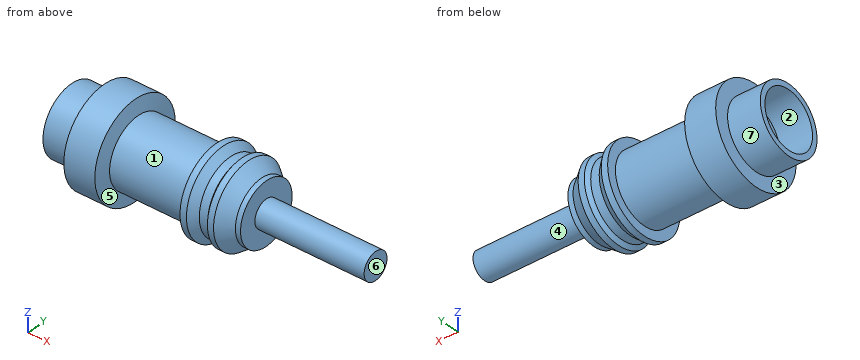
```python
from build123d import *

# Parameters (mm, degrees)
SKETCH_2_R          = 5.2
CUT_EXTRUDE_1_DEPTH = 6
SKETCH_3_R          = 2.5
EXTRUDE_1_DEPTH     = 20


with BuildPart() as part:
    # 草图1 → 旋转1 (revolve)
    with BuildSketch(Plane.XY):
        Polygon((0, 0), (0, 6.2), (6, 6.2), (6, 8.8), (11.676949671, 8.8), (12.2, 6.2), (26.523039375, 6.2), (26.523039375, 7.91006879), (27.695766684, 7.91006879), (29.059190298, 6.725292283), (30.614076117, 6.725292283), (31.1695333, 7.470731504), (32.294644919, 7.470731504), (34.759713658, 5.633908195), (35.7, 5.633908195), (35.7, 0), align=None)
    revolve(axis=Axis((35.7, 0, 0), (-1, 0, 0)))

    # 草图2 → 切除-拉伸1 (cut)
    with BuildSketch(Plane.ZY):
        with Locations(Location((0, 0, 0), (0, 0, 270))):
            Circle(SKETCH_2_R)
    extrude(amount=-CUT_EXTRUDE_1_DEPTH, mode=Mode.SUBTRACT)

    # 草图3 → 凸台-拉伸1 (add)
    with BuildSketch(Plane(origin=(35.7, 0, 0), x_dir=(0, 0, -1), z_dir=(1, 0, 0))):
        with Locations(Location((0, 0, 0), (0, 0, 90))):
            Circle(SKETCH_3_R)
    extrude(amount=EXTRUDE_1_DEPTH)


solid = part.part
```
Verification items for the finished model (mm, model axes). Face numbers are marked on the shaded views. A direction names the side the tool comes from. Give positions to 0.01 mm unless a question says otherwise; leave off trailing zeros. Order: outer loops, then holes, each group sorted by start corner. A loop starts at its lowest first (then second) coordinate and runs counter-clockwise, first axis right, second up. Notation, with made-up numbers: (71, 45) -> (111, 45) arc R16 cw to (111, 67) -> close; hole circle Ø4 at (-20.75, 61). An arc over 180 degrees is marked (long way). Use a Markdown table: item, result.
1) Material ranges on probe 1 along X at (y, z) = (6.75, 2); probe 2 along X at (y, z) = (7.25, -1.25); probe 3 along Z at (x, y) = (2.7, 0), recorded low to high.
Results:
| item | result |
|---|---|
| probe 1 | 6 to 12.03, 26.52 to 28.7, 30.85 to 32.87 |
| probe 2 | 6 to 11.97, 26.52 to 28.33, 31.08 to 32.45 |
| probe 3 | -6.2 to -5.2, 5.2 to 6.2 |
2) Depth check by flat-ended pin: pin 1 Ø4 at (y, z) = (6, 6) entering from -X; pin 2 Ø6 at (x, y) = (24, 2) entering from -Z; pin 3 Ø6 at (y, z) = (-6.5, 5) entering from +X. Enter the tip coordinate at first touch or a pass-through.
Results:
| item | result |
|---|---|
| pin 1 | x = 6 |
| pin 2 | z = -7.9 |
| pin 3 | x = 35.7 |
3) Mould release check, pull along X, two halves, no side actions. Record for the marked faces 1, 2 and 3: pulls with the +X half, pulls with the -X half, needs draft (parallel to the pull), parting line crosses it, or undercut.
Results:
| item | result |
|---|---|
| face 1 | undercut |
| face 2 | needs draft |
| face 3 | pulls with the -X half |
4) Section check B-B, the plane x = 22. Record the boundary of the cut face in (y, z), then the cut area to 3 significant figures.
Results:
| item | result |
|---|---|
| outline | circle Ø12.4 at (0, 0) |
| area | 121 mm² |
5) Tool access check on the marked faces 4, 5, 6 and 7. Record the directions out of +Z, -Z, +X, -X, +Y, -Y that give a thin tool (end or side, any length) a straight path to the whole face; none if there is none.
Results:
| item | result |
|---|---|
| face 4 | +X |
| face 5 | none |
| face 6 | +Z, -Z, +X, +Y, -Y |
| face 7 | -X |
6) Section check A-A, the plane x = 8.5. Record the boundary of the cut face in (y, z).
Results:
| item | result |
|---|---|
| outline | circle Ø17.6 at (0, 0) |
